```python
from build123d import *

# Parameters (mm, degrees)
SKETCH1_W                   = 88.9
SKETCH1_H                   = 53.975
BOSS_EXTRUDE1_DEPTH         = 20.6375
FILLET1_R                   = 7.9375
SKETCH3_W                   = 88.9
SKETCH3_H                   = 53.975
BOSS_EXTRUDE2_DEPTH         = 6.35
SHELL1_T                    = -6.35
SKETCH2_R                   = 7.14375
CUT_EXTRUDE1_DEPTH          = 47.625
F_16_0_177_DIAMETER_HOLE1_D = 4.4958
F_16_0_177_DIAMETER_HOLE2_D = 4.4958


with BuildPart() as part:
    # Sketch1 → Boss-Extrude1 (new body, symmetric)
    with BuildSketch(Plane.XY):
        Rectangle(SKETCH1_W, SKETCH1_H)
    extrude(amount=BOSS_EXTRUDE1_DEPTH, both=True)

    # Fillet1
    fillet1_edges = [part.edges().sort_by_distance(p)[0] for p in [
        (0, 26.9875, 20.6375),
        (0, -26.9875, 20.6375),
    ]]
    fillet(fillet1_edges, radius=FILLET1_R)

    # Sketch3 → Boss-Extrude2 (add)
    with BuildSketch(Plane(origin=(0, 0, -20.6375), x_dir=(-1, 0, 0), z_dir=(0, 0, -1))):
        Rectangle(SKETCH3_W, SKETCH3_H)
    extrude(amount=BOSS_EXTRUDE2_DEPTH)

    # Shell1
    shell1_openings = [part.faces().sort_by_distance(p)[0] for p in [
        (0, 0, -26.9875),
        (44.45, 0, 2.664636692),
        (-44.45, 0, 2.664636692),
    ]]
    offset(amount=SHELL1_T, openings=shell1_openings, kind=Kind.INTERSECTION)

    # Sketch2 → Cut-Extrude1 (cut)
    with BuildSketch(Plane.XY.offset(20.6375)):
        with Locations((-23.8125, 0)):
            Circle(SKETCH2_R)
        with Locations((23.8125, 0)):
            Circle(SKETCH2_R)
    extrude(amount=-CUT_EXTRUDE1_DEPTH, mode=Mode.SUBTRACT)

    # #16 (0.177) Diameter Hole1 (through all)
    with Locations(Plane(origin=(0, 26.9875, 0), x_dir=(1, 0, 0), z_dir=(0, 1, 0))):
        with Locations((-19.05, 11.1125), (-19.05, 20.6375)):
            Hole(F_16_0_177_DIAMETER_HOLE1_D / 2)

    # #16 (0.177) Diameter Hole2 (through all)
    with Locations(Plane.XY.offset(20.6375)):
        with Locations((0, -5), (0, 5)):
            Hole(F_16_0_177_DIAMETER_HOLE2_D / 2)


solid = part.part
```
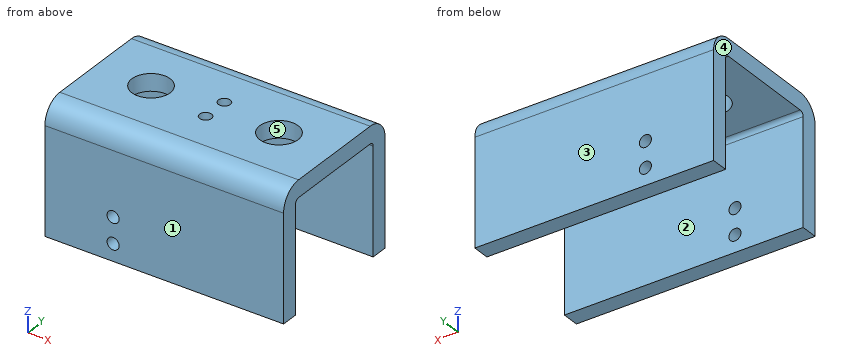
Here's how the part is built. I have some questions about the finished solid (model axes, mm). Face numbers are marked on the shaded views. A direction names the side the tool comes from. Coordinates: 2 decimals unless noted, no trailing zeros. Order: outer loops, then holes, each group sorted by start corner. A loop starts at its lowest first (then second) coordinate and runs counter-clockwise, first axis right, second up.
1) I need wall thicknesses on line 1 (Y direction, x = -23.5, z = -23); line 2 (X direction, y = 6.5, z = 17); line 3 (Z direction, x = -17, y = -6). Which ranges of each line are inside material? Lowest first, please.
2) Which directions (+Z, -Z, +X, -X, +Y, -Y) give clear straight access to the entire face, cutting with the end or side of a thin tool? Please do the marked faces 1 and 2.
3) Imagine slicing it at C-C on x = 0. State how many separate pieces and enclosed holes the cut face has, and give its area (3 significant figures).
4) Imagine slicing it at A-A on z = 0. List the corners of the cut face in (x, y) for me, and give its area (3 significant figures).
5) Will these pins go through, and if not, where does the flat tip stop? pin 1 (11.5 mm diameter, centred on x = 8.5, y = -6.5, fed in from -Z); pin 2 (6 mm diameter, centred on x = -19.05, z = -11.11, fed in from -Y).
6) Imagine slicing it at B-B on y = 0. List the corners of the cut face in (x, z) for me, and give its area (3 significant figures).
7) We'd pull the mould along Y, two halves only. Please class the marked faces 3, 4 and 5: +Y half, -Y half, draft (parallel to the pull), parting line (faces both ways), or undercut.
Response values:
1. line 1: y = -26.99 to -20.64, 20.64 to 26.99
1. line 2: x = -44.45 to -26.78, -20.85 to -1.67, 1.67 to 20.85, 26.78 to 44.45
1. line 3: z = 14.29 to 20.64
2. face 1: +Z, -Z, +X, -X, -Y
2. face 2: -Z, +X, -X
3. separate pieces: 3
3. enclosed holes: 0
3. area: 784 mm2
4. outline: (-44.45, -26.99) - (44.45, -26.99) - (44.45, -20.64) - (-44.45, -20.64) - close; (-44.45, 20.64) - (44.45, 20.64) - (44.45, 26.99) - (-44.45, 26.99) - close
4. area: 1,130 mm2
5. pin 1: stops at z = 14.29
5. pin 2: stops at y = -26.99
6. outline: (-44.45, 14.29) - (-30.96, 14.29) - (-30.96, 20.64) - (-44.45, 20.64) - close; (-16.67, 14.29) - (16.67, 14.29) - (16.67, 20.64) - (-16.67, 20.64) - close; (30.96, 14.29) - (44.45, 14.29) - (44.45, 20.64) - (30.96, 20.64) - close
6. area: 383 mm2
7. face 3: +Y half
7. face 4: draft
7. face 5: undercut
